```python
from build123d import *

# Parameters (mm, degrees)
SKETCH1_R           = 37.5
BOSS_EXTRUDE1_DEPTH = 5
SKETCH2_R           = 0.693
CUT_EXTRUDE1_DEPTH  = 6
SKETCH3_R           = 1.69
CUT_EXTRUDE2_DEPTH  = 6


with BuildPart() as part:
    # Sketch1 → Boss-Extrude1 (new body)
    with BuildSketch(Plane.XY):
        Circle(SKETCH1_R)
    extrude(amount=BOSS_EXTRUDE1_DEPTH)

    # Sketch2 → Cut-Extrude1 (cut, through all)
    with BuildSketch(Plane(origin=(0, 0, 0), x_dir=(-1, 0, 0), z_dir=(0, 0, -1))):
        Circle(SKETCH2_R)
    extrude(amount=-CUT_EXTRUDE1_DEPTH, mode=Mode.SUBTRACT)

    # Sketch3 → Cut-Extrude2 (cut, through all)
    with BuildSketch(Plane(origin=(0, 0, 0), x_dir=(-1, 0, 0), z_dir=(0, 0, -1))):
        with Locations((0, 32.5)):
            Circle(SKETCH3_R)
        with Locations((28.145825623, 16.25)):
            Circle(SKETCH3_R)
        with Locations((28.145825623, -16.25)):
            Circle(SKETCH3_R)
        with Locations((0, -32.5)):
            Circle(SKETCH3_R)
        with Locations((-28.145825623, -16.25)):
            Circle(SKETCH3_R)
        with Locations((-28.145825623, 16.25)):
            Circle(SKETCH3_R)
    extrude(amount=-CUT_EXTRUDE2_DEPTH, mode=Mode.SUBTRACT)


solid = part.part
```
Input: part model. Units: mm. Frame: model coordinates. Round coordinates to 2 decimals unless told otherwise and drop trailing zeros. Loops run counter-clockwise (first coordinate to the right, second up) from the corner with the lowest first, then second, coordinate; pieces in that order, holes last.
1) Section query B-B on z = 1.9. Return the cut outline in (x, y), plus the area to 3 significant figures.
Ans:
outline: circle Ø75 at (0, 0); hole circle Ø3.38 at (-28.15, -16.25); hole circle Ø3.38 at (-28.15, 16.25); hole circle Ø3.38 at (0, -32.5); hole circle Ø3.38 at (0, 32.5); hole circle Ø1.39 at (0, 0); hole circle Ø3.38 at (28.15, -16.25); hole circle Ø3.38 at (28.15, 16.25)
area: 4,360 mm2
2) Section query A-A on y = 32.5. Return the cut outline in (x, z), plus the area to 3 significant figures.
Ans:
outline: (-18.71, 0) - (-1.69, 0) - (-1.69, 5) - (-18.71, 5) - close; (1.69, 0) - (18.71, 0) - (18.71, 5) - (1.69, 5) - close
area: 170 mm2
3) Material intervals for line 1 (Y direction, x = 0, z = 3.95); line 2 (X direction, y = 32, z = 1.65); line 3 (Y direction, x = 10, z = 2.4), sorted ascending.
Ans:
line 1: y = -37.5 to -34.19, -30.81 to -0.69, 0.69 to 30.81, 34.19 to 37.5
line 2: x = -19.55 to -1.61, 1.61 to 19.55
line 3: y = -36.14 to 36.14
4) Section query D-D on x = -28. Return the cut outline in (y, z).
Ans:
outline: (-24.94, 0) - (-17.93, 0) - (-17.93, 5) - (-24.94, 5) - close; (-14.57, 0) - (14.57, 0) - (14.57, 5) - (-14.57, 5) - close; (17.93, 0) - (24.94, 0) - (24.94, 5) - (17.93, 5) - close
5) Pull-direction query (Y, two-part tool) for faces 1 (the cylindrical face through (-4.88, 37.18, 2.46)), 2 (the flat face through (-1, 1, 0)), 3 (the cylindrical face through (-1.61, -31.99, 2.46)); classes: released by +Y, released by -Y, zero draft, split by the parting line, or undercut.
Ans:
face 1: split by the parting line
face 2: zero draft
face 3: undercut
6) Section query C-C on y = 16.25. Return the cut outline in (x, z), plus the area to 3 significant figures.
Ans:
outline: (-33.8, 0) - (-29.84, 0) - (-29.84, 5) - (-33.8, 5) - close; (-26.46, 0) - (26.46, 0) - (26.46, 5) - (-26.46, 5) - close; (29.84, 0) - (33.8, 0) - (33.8, 5) - (29.84, 5) - close
area: 304 mm2
7) Pin query (flat end, axial travel): pin 1 (1 mm diameter, centred on y = -29, z = 3.5, fed in from -X); pin 2 (2 mm diameter, centred on x = 21, z = 1.5, fed in from +Y); pin 3 (1.5 mm diameter, centred on y = -10, z = 3, fed in from -X). Return the tip coordinate at first contact, or that it passes through.
Ans:
pin 1: stops at x = -24.37
pin 2: stops at y = 31.72
pin 3: stops at x = -36.34
